Design review of the part shown in the three views and the two pictorial views. Dimensions are in mm from the part's minimum x, y and z. A direction names the side the tool comes from. Round coordinates to 2 decimals unless told otherwise and drop trailing zeros. Write each loop counter-clockwise with the first axis right and the second up, starting at its lowest first coordinate (ties: lowest second). Pieces come first, ordered by that corner, then holes. Notation, with made-up numbers: (49, -17) - (76, -17) arc R26 ccw to (76, 14) - close; hole circle Ø9 at (-13.5, 79.25). An arc over 180 degrees is marked (long way). Use one line per item in the form item = value.
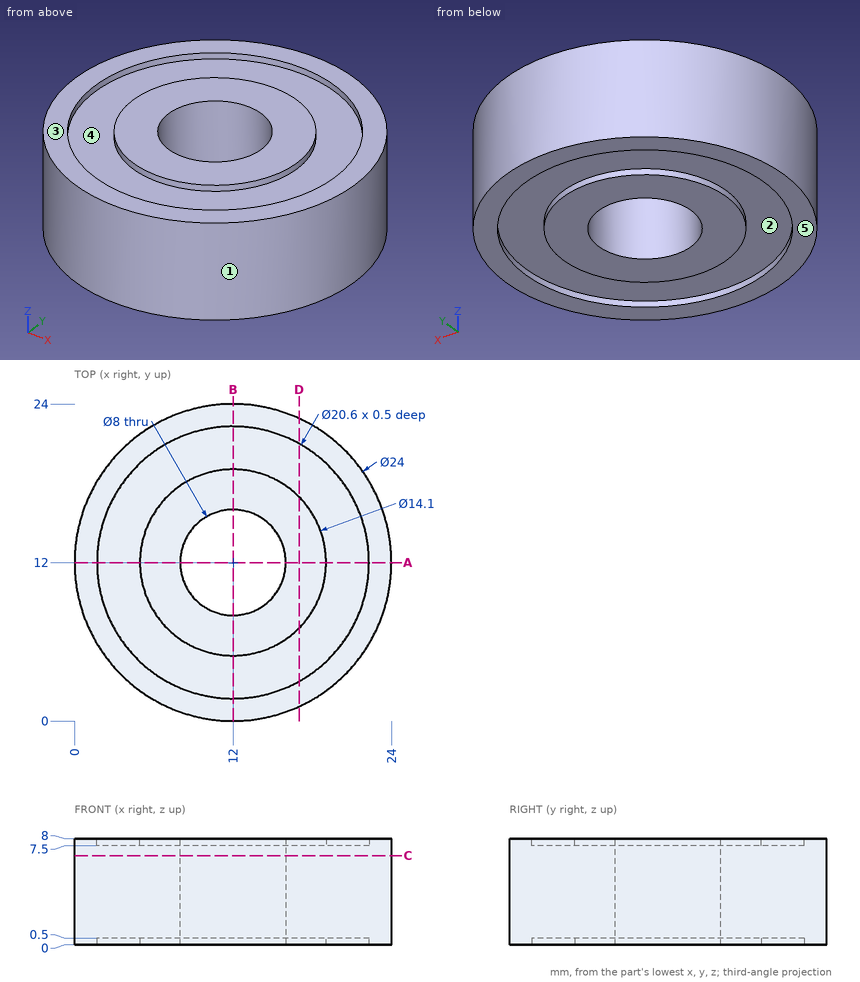
Q1. For P1, Ø2, axis at y = 17.5, z = 1.5, coming from the -X side; P2, Ø6.5, axis at x = 12, y = 12, coming from the -Z side; P3, Ø1.5, axis at y = 7, z = 6, coming from the +X side, all flat-tipped, find the tip position at first contact; note any pin that passes through.
Calculated:
P1 = 0.88
P2 = through
P3 = 23.22
Q2. We need section C-C on z = 6.75. Write out the cut boundary in (x, y).
Calculated:
outline = circle Ø24 at (12, 12); hole circle Ø8 at (12, 12)
Q3. Draft analysis for pull direction Y (two halves, no side actions). For the marked faces 1, 2 and 3, state which applies: released by +Y, released by -Y, zero draft, split by the parting line, or undercut.
Calculated:
face_1 = split by the parting line
face_2 = undercut
face_3 = zero draft
Q4. To check wall thickness, follow line 1 along Y through (x, z) = (12, 0.4); line 2 along Y through (x, z) = (12, 4.5); line 3 along Z through (x, y) = (4.25, 10.5). State the ranges of each line that lie inside material, in increasing order. Write a range as from..to.
Calculated:
line_1 = 0..1.7, 4.95..8, 16..19.05, 22.3..24
line_2 = 0..8, 16..24
line_3 = 0.5..7.5
Q5. We need section D-D on x = 17. Write out the cut boundary in (y, z) (3 decimals), then the cut area to 3 significant figures.
Calculated:
outline = (1.091, 0) - (2.995, 0) - (2.995, 0.5) - (7.03, 0.5) - (7.03, 0) - (16.97, 0) - (16.97, 0.5) - (21.005, 0.5) - (21.005, 0) - (22.909, 0) - (22.909, 8) - (21.005, 8) - (21.005, 7.5) - (16.97, 7.5) - (16.97, 8) - (7.03, 8) - (7.03, 7.5) - (2.995, 7.5) - (2.995, 8) - (1.091, 8) - close
area = 166 mm2
Q6. Machinability: for the marked faces 4 and 5, which of the approach directions +Z, -Z, +X, -X, +Y, -Y give a long, thin tool a straight path to every point of the face, cutting with its end or side? Answer none if there is none.
Calculated:
face_4 = +Z
face_5 = -Z, +X, -X, +Y, -Y
Q7. We need section A-A on y = 12. Write out the cut boundary in (x, z), then the cut area to 4 significant figures.
Calculated:
outline = (0, 0) - (1.7, 0) - (1.7, 0.5) - (4.95, 0.5) - (4.95, 0) - (8, 0) - (8, 8) - (4.95, 8) - (4.95, 7.5) - (1.7, 7.5) - (1.7, 8) - (0, 8) - close; (16, 0) - (19.05, 0) - (19.05, 0.5) - (22.3, 0.5) - (22.3, 0) - (24, 0) - (24, 8) - (22.3, 8) - (22.3, 7.5) - (19.05, 7.5) - (19.05, 8) - (16, 8) - close
area = 121.5 mm2
